from build123d import *

# Parameters (mm, degrees)
F0_W           = 152.4
F0_H           = 101.6
F1_DEPTH       = 101.6
F3_DEPTH       = 101.601
F5_DEPTH       = 88.9
F7_D           = 10.0838
F7_CSINK_D     = 19.8374
F7_CSINK_ANGLE = 82
F9_D           = 13.49248


with BuildPart() as f1:
    # F0 (on Front) → F1 (new body)
    with BuildSketch(Plane.XZ):
        with Locations((76.2, 50.8)):
            Rectangle(F0_W, F0_H)
    extrude(amount=F1_DEPTH)

    # F2 (on face) → F3 (cut, through all)
    with BuildSketch(Plane.XZ.offset(101.6)):
        Polygon((0, 50.8), (152.4, 76.2), (152.4, 101.6), (0, 101.6), align=None)
    extrude(amount=-F3_DEPTH, mode=Mode.SUBTRACT)

    # F4 (on face) → F5 (cut)
    with BuildSketch(Plane.XZ.offset(101.6)):
        Polygon((0, 37.9248193109), (0, 0), (152.4, 0), (152.4, 63.3248193109), align=None)
    extrude(amount=-F5_DEPTH, mode=Mode.SUBTRACT)

    # F7 (through all)
    with Locations(Plane.XZ.offset(12.7)):
        with Locations((25.4, 19.05), (127, 19.05)):
            CounterSinkHole(F7_D / 2, F7_CSINK_D / 2, counter_sink_angle=F7_CSINK_ANGLE)

    # F9 (through all)
    with Locations(Plane(origin=(-8.2378378378, 0, 49.427027027), x_dir=(0.9863939238, 0, 0.1643989873), z_dir=(-0.1643989873, 0, 0.9863939238))):
        with Locations((124.7536368247, -50.8), (48.5536368247, -50.8)):
            Hole(F9_D / 2)


solid = f1.part
Geometry: final body of the model. Coordinates: model frame, mm. A direction names the side the tool comes from. Give positions to 0.01 mm unless a question says otherwise; leave off trailing zeros. Loops run counter-clockwise (first coordinate to the right, second up) from the corner with the lowest first, then second, coordinate; pieces in that order, holes last. Notation, with made-up numbers: M 28,36 L 78,36 A31 cw 78,68 Z; hole C -1,57 d8. An arc over 180 degrees is marked long. Put each result on its own line as item: value. Start each with the question number.
1) Cut plane B-B (x = 25.4). Output: boundary loops of the cut face in (y, z).
2) Cut plane A-A (z = 19.05). Output: boundary loops of the cut face in (x, y), then the cut area to 3 significant figures.
3) Cut plane C-C (y = -53). Output: boundary loops of the cut face in (x, z), then the cut area to 3 significant figures.
4) Access query for faces 5 (the flat face through (77.267, -57.772, 50.803)), 6 (the cylindrical face through (112.3, -45.11, 62.99)). Directions: +Z, -Z, +X, -X, +Y, -Y. A direction counts if a zero-diameter tool reaches every point of the face in a straight line with its end or side. Return the directions, or none.
5) Pull-direction query (X, two-part tool) for faces 1 (the flat face through (75.13, -51.51, 63.32)), 2 (the flat face through (75, -12.7, 25)), 3 (the cylindrical face through (122.19, -3.5, 20.56)), 4 (the cylindrical face through (22.69, -3.5, 23.3)); classes: pulls with the +X half, pulls with the -X half, needs draft (parallel to the pull), parting line crosses it, or undercut.
6) Contact query for flat-ended pins moving along their axis: pin 1 (1 mm diameter, centred on x = 127.5, y = -91, fed in from +Z); pin 2 (3 mm diameter, centred on x = 126.5, y = -51, fed in from -Z); pin 3 (6 mm diameter, centred on x = 127, z = 19, fed in from -Y); pin 4 (11.5 mm diameter, centred on x = 25.4, z = 19.05, fed in from -Y). Output: stop coordinate, or through.
7) Ray query, line 1 along X through (y, z) = (-3, 19); line 2 along X through (y, z) = (-10.5, 21); line 3 along Y through (x, z) = (24, 7). Return the intervals inside material, ascending.
8) Cut plane D-D (y = -19.5). Output: boundary loops of the cut face in (x, z).
Verdict:
1. outline: M -101.6,42.16 L -12.7,42.16 L -12.7,28.97 L -7.09,24.09 L 0,24.09 L 0,55.03 L -101.6,55.03 Z; M -12.7,0 L 0,0 L 0,14.01 L -7.09,14.01 L -12.7,9.13 Z
2. outline: M 0,-12.7 L 15.48,-12.7 L 20.36,-7.09 L 20.36,0 L 0,0 Z; M 30.44,-7.09 L 35.32,-12.7 L 117.08,-12.7 L 121.96,-7.09 L 121.96,0 L 30.44,0 Z; M 132.04,-7.09 L 136.92,-12.7 L 152.4,-12.7 L 152.4,0 L 132.04,0 Z
2. area: 1,620 mm2
3. outline: M 0,37.92 L 35.45,43.83 L 33.36,56.36 L 0,50.8 Z; M 45.95,58.46 L 48.03,45.93 L 110.62,56.36 L 108.53,68.89 Z; M 121.11,70.98 L 123.2,58.46 L 152.4,63.32 L 152.4,76.2 Z
3. area: 1,640 mm2
4. face 5: -Z, +X, -Y
4. face 6: none
5. face 1: pulls with the -X half
5. face 2: needs draft
5. face 3: undercut
5. face 4: undercut
6. pin 1: z = 72.13
6. pin 2: z = 58.76
6. pin 3: through
6. pin 4: y = -7.9
7. line 1: 0 to 20.36, 30.44 to 121.96, 132.04 to 152.4
7. line 2: 0 to 17.63, 33.17 to 119.23, 134.77 to 152.4
7. line 3: -12.7 to 0
8. outline: M 0,37.92 L 152.4,63.32 L 152.4,76.2 L 0,50.8 Z
